CAD build for the part. Positions are in the model's coordinates, mm. A direction names the side the tool comes from. Coordinates: 2 decimals unless noted, no trailing zeros. Loops run counter-clockwise (first coordinate to the right, second up) from the corner with the lowest first, then second, coordinate; pieces in that order, holes last. Notation, with made-up numbers: (6, -35) -> (22, -35) arc R12 ccw to (22, -31) -> close; hole circle Ø3 at (-19, 58). An arc over 180 degrees is marked (long way). Write each question's results on one line, items separated by ' | '.
```python
from build123d import *

# Parameters (mm, degrees)
F1_DEPTH = 17.4625
F2_T     = -3.175
F0_R     = 3.175
F0_R_2   = 3.25
F3_DEPTH = 6.35
F4_R     = 1
F4_R_2   = 1.25
F5_DEPTH = 14.2875
F4_R_3   = 6.45
F6_DEPTH = 3.176


# Not quite as in the source:
# - a feature names something its author has since deleted; it is built from what else it names


with BuildPart() as f1:
    # F0 (on Top) → F1 (new body)
    with BuildSketch(Plane.XY):
        Polygon((-32.7674517391, -39.2625403754), (13.6125482609, -39.2625403754), (13.6125482609, -31.3625403754), (21.5125482609, -31.3625403754), (32.3125482609, -31.3625403754), (37.0125482609, -31.3625403754), (37.0125482609, -15.3529706535), (29.1460849644, 6.2599596246), (20.8971929933, 11.0224596246), (0, 23.0874596246), (-32.7674517391, 23.0874596246), (-32.7674517391, -29.7375403754), align=None)
    extrude(amount=-F1_DEPTH)

    # F2
    f2_openings = [f1.faces().sort_by_distance(p)[0] for p in [
        (-2.028392, -9.399027, 0),
    ]]
    offset(amount=F2_T, openings=f2_openings, kind=Kind.INTERSECTION)

    # F0 (on Top) → F3 (join)
    with BuildSketch(Plane.XY):
        with BuildLine():
            Line((-45.4674517391, -39.2625403754), (-32.7674517391, -39.2625403754))
            Line((-32.7674517391, -39.2625403754), (-32.7674517391, -29.7375403754))
            Line((-32.7674517391, -29.7375403754), (-45.4674517391, -29.7375403754))
            ThreePointArc((-45.4674517391, -29.7375403754), (-50.2299517391, -34.5000403754), (-45.4674517391, -39.2625403754))
        make_face()
        with Locations((-45.4674517391, -34.5000403754)):
            Circle(F0_R, mode=Mode.SUBTRACT)
        with BuildLine():
            Line((27.2471929933, 22.0209822527), (20.8971929933, 11.0224596246))
            Line((20.8971929933, 11.0224596246), (29.1460849644, 6.2599596246))
            Line((29.1460849644, 6.2599596246), (35.4960849644, 17.2584822527))
            ThreePointArc((35.4960849644, 17.2584822527), (33.7528889788, 23.7641782382), (27.2471929933, 22.0209822527))
        make_face()
        with Locations((31.3716389788, 19.6397322527)):
            Circle(F0_R, mode=Mode.SUBTRACT)
        with BuildLine():
            Line((32.3125482609, -31.3625403754), (21.5125482609, -31.3625403754))
            Line((21.5125482609, -31.3625403754), (21.5125482609, -39.2625403754))
            ThreePointArc((21.5125482609, -39.2625403754), (26.9125482609, -44.6625403754), (32.3125482609, -39.2625403754))
            Line((32.3125482609, -39.2625403754), (32.3125482609, -31.3625403754))
        make_face()
        with Locations((26.9125482609, -39.2625403754)):
            Circle(F0_R_2, mode=Mode.SUBTRACT)
    extrude(amount=-F3_DEPTH)

    # F4 (on face) → F5 (join, through all)
    with BuildSketch(Plane.XY.offset(-14.2875)):
        with Locations((26.905224515, -13.3725403754)):
            Circle(F4_R)
        with Locations((18.055224515, -0.9225403754)):
            Circle(F4_R_2)
    extrude(amount=F5_DEPTH)

    # F4 (on face) → F6 (cut, through all)
    with BuildSketch(Plane.XY.offset(-14.2875)):
        with Locations((-3.9174517391, 5.3074596246)):
            Circle(F4_R_3)
    extrude(amount=-F6_DEPTH, mode=Mode.SUBTRACT)


solid = f1.part
```
Q1. Cut at C-C on z = -12. Write the cut outline in (x, y).
Results are:
outline: (-32.77, -39.26) -> (13.61, -39.26) -> (13.61, -31.36) -> (37.01, -31.36) -> (37.01, -15.35) -> (29.15, 6.26) -> (0, 23.09) -> (-32.77, 23.09) -> close; circle Ø2.5 at (18.06, -0.92); circle Ø2 at (26.91, -13.37); hole (-29.59, -36.09) -> (10.44, -36.09) -> (10.44, -28.19) -> (33.84, -28.19) -> (33.84, -15.91) -> (26.56, 4.09) -> (-0.85, 19.91) -> (-29.59, 19.91) -> close
Q2. Pull direction X, two halves, no side cores. Call faces 6 (the flat face through (-39, -29.738, -3)), 7 (the flat face through (30.249, -6.052, -7.044)), 8 (the flat face through (-10, -36.088, -7)), 9 (the flat face through (32.277, 11.682, -3.131)): +X half, -X half, draft (parallel to the pull), parting line (faces both ways), or undercut.
Results are:
face 6: draft | face 7: undercut | face 8: undercut | face 9: +X half
Q3. Wall check: L1, parallel to X at y = 15, z = -2; L2, parallel to Y at x = -23, z = -12.5; L3, parallel to X at y = -13, z = -8.25. Give the ranges that are in metal, low to high. Write a range as from..to.
Results are:
L1: -32.77..-29.59, 7.66..14.01, 23.19..34.19 | L2: -39.26..-36.09, 19.91..23.09 | L3: -32.77..-29.59, 25.98..27.83, 32.78..36.16
Q4. Which spindle directions (+Z, -Z, +X, -X, +Y, -Y) get a long thin tool onto all of the face, cutting with end or side? Do faces 1 (the flat face through (32.313, -35, -3)), 2 (the flat face through (24.117, 16.599, -3.131)), 3 (the flat face through (13.613, -35, -9)), 4 (the flat face through (33.838, -22, -7)), 5 (the flat face through (-16, 23.087, -9)). Say none if no direction does.
Results are:
face 1: +Z, -Z, +X, -Y | face 2: +Z, -Z, +Y | face 3: +Z, -Z, -Y | face 4: +Z | face 5: +Z, -Z, -X, +Y
Q5. Cut at D-D on x = -15.5. Write the cut outline in (y, z), and give its area (3 significant figures).
Results are:
outline: (-39.26, -17.46) -> (23.09, -17.46) -> (23.09, 0) -> (19.91, 0) -> (19.91, -14.29) -> (-36.09, -14.29) -> (-36.09, 0) -> (-39.26, 0) -> close | area: 289 mm^2
Q6. Cut at A-A on z = -5.25. Give the number of separate pieces and of enclosed holes in the cut face, and give its area (3 significant figures).
Results are:
separate pieces: 3 | enclosed holes: 4 | area: 1,100 mm^2
Q7. Drop flat-ended pins along their axis: pin 1 (7.5 mm diameter, centred on x = 26.91, y = -39.26, fed in from +Z); pin 2 (8.5 mm diameter, centred on x = 29, y = -39, fed in from -Z); pin 3 (3 mm diameter, centred on y = -34.5, z = -3, fed in from +X); pin 4 (4 mm diameter, centred on y = -32, z = -4, fed in from -X). Give the stop position or say it passes through.
Results are:
pin 1: z = 0 | pin 2: z = -6.35 | pin 3: x = 32.31 | pin 4: x = -50.2
Q8. Cut at B-B on y = -22.5. Write the cut outline in (x, z).
Results are:
outline: (-32.77, -17.46) -> (37.01, -17.46) -> (37.01, 0) -> (33.84, 0) -> (33.84, -14.29) -> (-29.59, -14.29) -> (-29.59, 0) -> (-32.77, 0) -> close
